Verification items for the finished model (mm, model axes). Face numbers are marked on the shaded views. A direction names the side the tool comes from. Give positions to 0.01 mm unless a question says otherwise; leave off trailing zeros. Loops run counter-clockwise (first coordinate to the right, second up) from the corner with the lowest first, then second, coordinate; pieces in that order, holes last. Notation, with made-up numbers: M -7,65 L 22,65 A30 cw 22,98 Z; hole C 26.25,40.5 d6. An arc over 180 degrees is marked long. Answer in a Markdown table with one row per item.
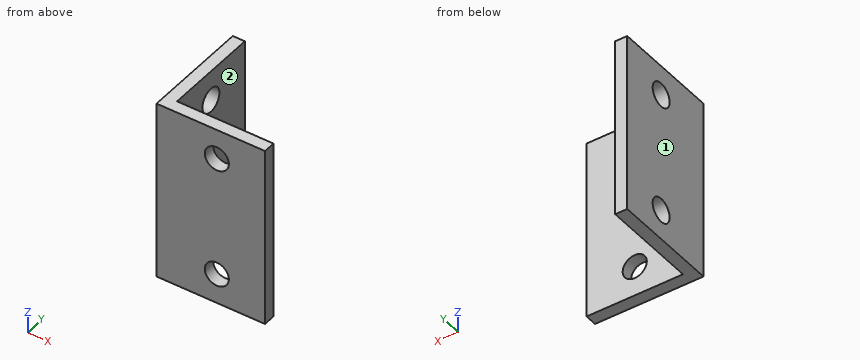
```python
from build123d import *

# Parameters (mm, degrees)
F1_DEPTH = 15
F2_R     = 1
F3_DEPTH = 1
F4_R     = 1
F5_DEPTH = 1


with BuildPart() as f1:
    # F0 (on Top) → F1 (new body)
    with BuildSketch(Plane.XY):
        Polygon((0, 9), (0, 0), (9, 0), (9, 1), (1, 1), (1, 9), align=None)
    extrude(amount=F1_DEPTH)

    # F2 (on face) → F3 (cut, through all)
    with BuildSketch(Plane.XZ):
        with Locations((5, 12.5)):
            Circle(F2_R)
        with Locations((5, 2.5)):
            Circle(F2_R)
    extrude(amount=-F3_DEPTH, mode=Mode.SUBTRACT)

    # F4 (on face) → F5 (cut, through all)
    with BuildSketch(Plane(origin=(0, 0, 0), x_dir=(0, -1, 0), z_dir=(-1, 0, 0))):
        with Locations((-5, 12.5)):
            Circle(F4_R)
        with Locations((-5, 2.5)):
            Circle(F4_R)
    extrude(amount=-F5_DEPTH, mode=Mode.SUBTRACT)


solid = f1.part
```
Item 1: Go/stop test with flat-tipped pins: pin 1 (1 mm diameter, centred on x = 5.5, z = 3, fed in from +Y); pin 2 (3 mm diameter, centred on y = 5, z = 2.5, fed in from +X). Record where each tip stops, or that it passes through.
Reported:
| item | result |
|---|---|
| pin 1 | stops at y = 1 |
| pin 2 | stops at x = 1 |
Item 2: Sectioned sample at A-A (y = 5). Record the cut outline in (x, z), and give its area (3 significant figures).
Reported:
| item | result |
|---|---|
| outline | M 0,0 L 1,0 L 1,1.5 L 0,1.5 Z; M 0,3.5 L 1,3.5 L 1,11.5 L 0,11.5 Z; M 0,13.5 L 1,13.5 L 1,15 L 0,15 Z |
| area | 11.0 mm^2 |
Item 3: Tool access check on the marked faces 1 and 2. Record the directions out of +Z, -Z, +X, -X, +Y, -Y that give a thin tool (end or side, any length) a straight path to the whole face; none if there is none.
Reported:
| item | result |
|---|---|
| face 1 | +Z, -Z, -X, +Y, -Y |
| face 2 | +Z, -Z, +X, +Y |
Item 4: Sectioned sample at C-C (z = 12.5). Record the cut outline in (x, y).
Reported:
| item | result |
|---|---|
| outline | M 0,0 L 4,0 L 4,1 L 1,1 L 1,4 L 0,4 Z; M 0,6 L 1,6 L 1,9 L 0,9 Z; M 6,0 L 9,0 L 9,1 L 6,1 Z |
Item 5: Scan lines: L1, parallel to Z at x = 0.5, y = 5; L2, parallel to Y at x = 6.5, z = 2.75. Record each from-to range of solid material in increasing order. Write a range as [from, to].
Reported:
| item | result |
|---|---|
| L1 | z = [0, 1.5], [3.5, 11.5], [13.5, 15] |
| L2 | y = [0, 1] |
Item 6: Sectioned sample at D-D (y = 3.5). Record the cut outline in (x, z).
Reported:
| item | result |
|---|---|
| outline | M 0,0 L 1,0 L 1,15 L 0,15 Z |
